Print and shaded views of the part. All mm, measured from the part's lowest x, y and z. A direction names the side the tool comes from. Give positions to 0.01 mm unless a question says otherwise; leave off trailing zeros. Write each loop counter-clockwise with the first axis right and the second up, starting at its lowest first coordinate (ties: lowest second). Pieces come first, ordered by that corner, then holes. Notation, with made-up numbers: (60.5, -16) -> (76.5, -16) arc R25 ccw to (76.5, -3) -> close; hole circle Ø5 at (-26, 14). An arc over 180 degrees is marked (long way). Put each result on its own line as item: value.
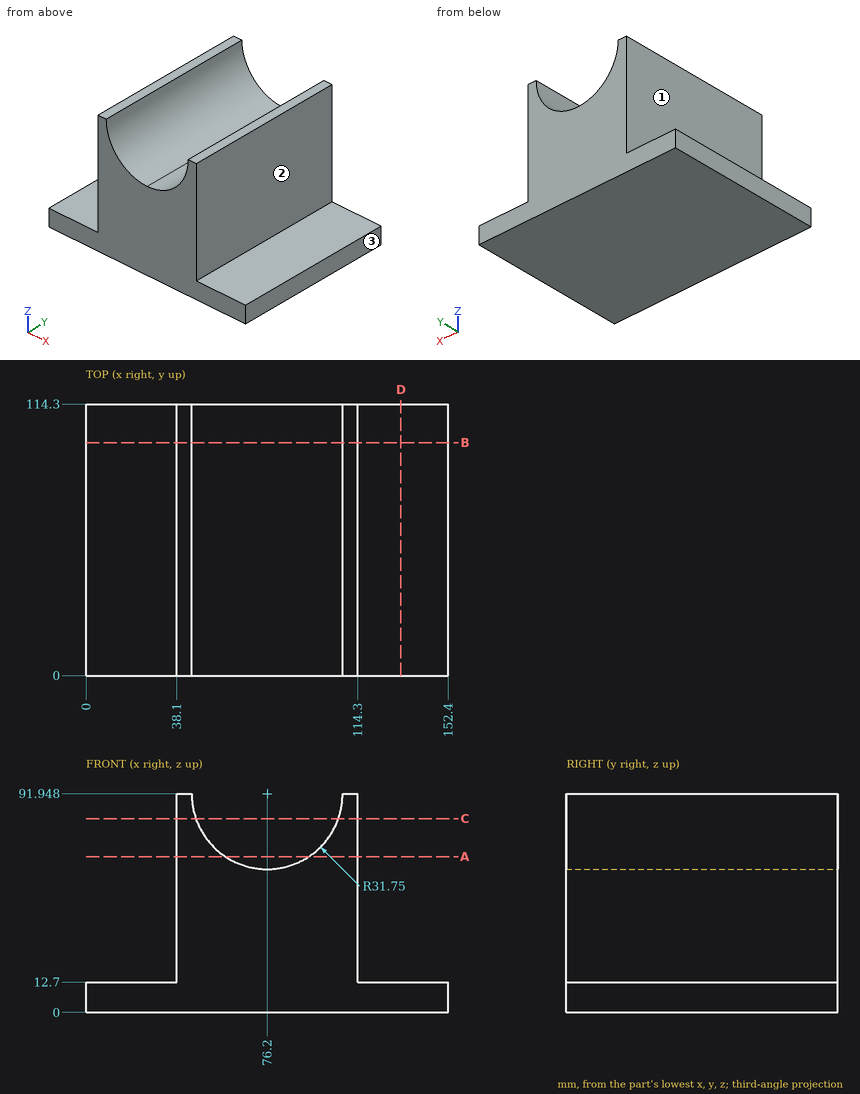
1) Slice it at C-C (z = 81.5). Write the cut outline in (x, y), plus the area to 3 significant figures.
Filled sheet:
outline: (38.1, 0) -> (46.22, 0) -> (46.22, 114.3) -> (38.1, 114.3) -> close; (106.18, 0) -> (114.3, 0) -> (114.3, 114.3) -> (106.18, 114.3) -> close
area: 1,860 mm2
2) Wall check: L1, parallel to X at y = 41, z = 13.5; L2, parallel to X at y = 96.5, z = 63; L3, parallel to X at y = 37, z = 80. Give the ranges that are in metal, low to high.
Filled sheet:
L1: 38.1 to 114.3
L2: 38.1 to 63.16, 89.24 to 114.3
L3: 38.1 to 46.78, 105.62 to 114.3
3) Slice it at A-A (z = 65.5). Write the cut outline in (x, y).
Filled sheet:
outline: (38.1, 0) -> (58.63, 0) -> (58.63, 114.3) -> (38.1, 114.3) -> close; (93.77, 0) -> (114.3, 0) -> (114.3, 114.3) -> (93.77, 114.3) -> close
4) Tool access for the marked faces 1, 2 and 3: list every direction of +Z, -Z, +X, -X, +Y, -Y with a clear straight run to the whole face (end or side of a thin tool).
Filled sheet:
face 1: +Z, -X, +Y, -Y
face 2: +Z, +X, +Y, -Y
face 3: +Z, -Z, +X, +Y, -Y
5) Slice it at D-D (x = 132.5). Write the cut outline in (y, z).
Filled sheet:
outline: (0, 0) -> (114.3, 0) -> (114.3, 12.7) -> (0, 12.7) -> close
6) Pin check, flat tips, straight feed: pin 1 (1 mm diameter, centred on y = 61, z = 24.5, fed in from +X); pin 2 (6 mm diameter, centred on x = 125.5, y = 50.5, fed in from +Z); pin 3 (8 mm diameter, centred on y = 85, z = 39.5, fed in from -X). Stop position of each tip, or through.
Filled sheet:
pin 1: x = 114.3
pin 2: z = 12.7
pin 3: x = 38.1
7) Slice it at B-B (y = 98). Write the cut outline in (x, z), plus the area to 3 significant figures.
Filled sheet:
outline: (0, 0) -> (152.4, 0) -> (152.4, 12.7) -> (114.3, 12.7) -> (114.3, 91.95) -> (107.95, 91.95) arc R31.75 cw to (76.2, 60.2) arc R31.75 cw to (44.45, 91.95) -> (38.1, 91.95) -> (38.1, 12.7) -> (0, 12.7) -> close
area: 6,390 mm2
